Autodesk Inventor part; units mm, degrees
ref_plane "YZ Plane" through (0, 0, 0) normal (1, 0, 0) x (0, 1, 0)
ref_plane "XZ Plane" through (0, 0, 0) normal (0, 1, 0) x (-1, 0, 0)
ref_plane "XY Plane" through (0, 0, 0) normal (0, 0, 1) x (1, 0, 0)
sketch "Skizze21" plane through (0, 0, 0) normal (0, 0, 1) x (1, 0, 0)
  line L0 (0, 0) -> (20, 0)
  line L1 (20, 0) -> (20, -6.5)
  line L2 (20, -6.5) -> (0, -6.5)
  line L3 (0, -6.5) -> (0, 0)
  dimension "d73" = 6.5
  dimension "d74" = 20
extrude "Extrusion16" add sketch "Skizze21" along normal mid plane 9
sketch "Skizze24" plane through (0, 0, 0) normal (0, 0, 1) x (1, 0, 0)
  line L0 (4.5, -2.3) -> (4.5, 0)
  line L1 (4.5, 0) -> (0, 0)
  line L2 (0, 0) -> (0, -2.5)
  line L3 (20, 0) -> (0, 0)
  line L4 (0, 0) -> (0, -6.5)
  line L5 (4.5, -2.3) -> (0, -2.5)
  dimension "d92" = 4.5
  dimension "d101" = 2.3
  dimension "d102" = 2.5
extrude "Extrusion19" cut sketch "Skizze24" along normal mid plane 16.5
sketch "Skizze23" plane through (0, 0, 4.5) normal (0, 1, 0) x (1, 0, 0)
  line L0 (0, 4.5) -> (36.014, 4.5) construction
  circle A0 centre (11, 4.5) radius 4
  line L1 (0, 0) -> (0, 9)
  line L2 (4.5, 9) -> (4.5, 0)
  dimension "d87" = 8
  dimension "d96" = 6.5
extrude "Extrusion18" add sketch "Skizze23" along normal blind 5
chamfer "Fasen2" distance 3 angle 45 1 edges at (0, -6.5, 0)
fillet "Rundung11" radius 2 2 edges at (0, -3, 4.5) (0, -3, -4.5)
sketch "Skizze25" plane through (20, -6.5, 4.5) normal (1, 0, 0) x (0, 0, -1)
  line L0 (9, 6.5) -> (0, 6.5)
  line L1 (9, 6.5) -> (9, 0)
  circle A0 centre (4.5, 3) radius 3
  line L2 (4.5, 6.5) -> (4.5, 0) construction
  line L3 (9, 0) -> (0, 0)
  line L4 (1.5, 3) -> (1.5, 0)
  line L5 (7.5, 0) -> (7.5, 3)
  dimension "d106" = 6
extrude "Extrusion20" cut sketch "Skizze25" against normal blind 4
properties part number "P_handle"
Can you work these out from the model? Positions are in its coordinate system, mm. A direction names the side the tool comes from. Coordinates: 2 decimals unless noted, no trailing zeros. Loops run counter-clockwise (first coordinate to the right, second up) from the corner with the lowest first, then second, coordinate; pieces in that order, holes last. Notation, with made-up numbers: M 71.25,89 L 108.25,89 A27 cw 108.25,128 Z; hole C 65.25,-33.5 d8. An arc over 180 degrees is marked long. Put each result on its own line as item: value. Start each with the question number.
(1) I need wall thicknesses on probe 1 along Y at (x, z) = (18.5, 4); probe 2 along X at (y, z) = (-1.5, -2); probe 3 along X at (y, z) = (-5.5, -1.75). Which ranges of each line are inside material? Lowest first, please.
(2) Imagine slicing it at A-A on x = 18.75. List the corners of the cut face in (y, z) for me, and give its area (3 significant figures).
(3) Imagine slicing it at C-C on y = -4.25. List the corners of the cut face in (x, z) for me, and give its area (3 significant figures).
(4) Which directions (+Z, -Z, +X, -X, +Y, -Y) give clear straight access to the entire face, cutting with the end or side of a thin tool? Please do faces 1 (the face through (7.8, 2.5, -2.4)), 2 (the face through (20, -1, -2)), 3 (the face through (18, -5, 3)).
(5) Imagine slicing it at B-B on z = 0. List the corners of the cut face in (x, y) for me.
(6) Imagine slicing it at D-D on x = 11. List the corners of the cut face in (y, z) for me.
(7) Will these pins go through, and if not, where does the flat tip stop? pin 1 Ø4 at (y, z) = (3, 2.5) entering from -X; pin 2 Ø1.8 at (y, z) = (-1, -0.5) entering from -X; pin 3 Ø5 at (y, z) = (-3.5, 0) entering from +X.
(8) We'd pull the mould along Z, two halves only. Please class faces 4 (the face through (4.5, -1, 0)), 5 (the face through (16, -3, 0)), 6 (the face through (11, -3, 4.5)): +Z half, -Z half, draft (parallel to the pull), parting line (faces both ways), or undercut.
Worked answers:
1. probe 1: y = -6.5 to 0
1. probe 2: x = 4.5 to 16
1. probe 3: x = 2 to 16
2. outline: M -6.5,-4.5 L 0,-4.5 L 0,4.5 L -6.5,4.5 L -6.5,3 L -3.5,3 A3 cw -3.5,-3 L -6.5,-3 Z
2. area: 26.4 mm2
3. outline: M 0.75,-4.06 A2 ccw 2,-4.5 L 20,-4.5 L 20,-3 L 16,-3 L 16,3 L 20,3 L 20,4.5 L 2,4.5 A2 ccw 0.75,4.06 Z
3. area: 149 mm2
4. face 1: +Y
4. face 2: +Z, -Z, +X, +Y, -Y
4. face 3: +X, -Y
5. outline: M 0,-3.5 L 3,-6.5 L 16,-6.5 L 16,-0.5 L 20,-0.5 L 20,0 L 15,0 L 15,5 L 7,5 L 7,0 L 4.5,0 L 4.5,-2.3 L 0,-2.5 Z
6. outline: M -6.5,-4.5 L 0,-4.5 L 0,-4 L 5,-4 L 5,4 L 0,4 L 0,4.5 L -6.5,4.5 Z
7. pin 1: stops at x = 7.03
7. pin 2: stops at x = 4.5
7. pin 3: stops at x = 16
8. face 4: draft
8. face 5: undercut
8. face 6: +Z half
